```python
from build123d import *

# Parameters (mm, degrees)
SKETCH1_W           = 50.8
SKETCH1_H           = 6.6675
BOSS_EXTRUDE1_DEPTH = 44.45
CHAMFER1_SIZE       = 2.54
CHAMFER2_SIZE       = 2.54
SKETCH2_R           = 11.176
CUT_EXTRUDE1_DEPTH  = 44.45


with BuildPart() as part:
    # Sketch1 → Boss-Extrude1 (new body)
    with BuildSketch(Plane(origin=(0, 0, 0), x_dir=(1, 0, 0), z_dir=(0, 1, 0))):
        Polygon((0, 22.5425), (0, 15.875), (0, 9.2075), (0, 0), (41.275, 0), (41.275, 31.75), (0, 31.75), align=None)
        with Locations((-25.4, 19.20875)):
            Rectangle(SKETCH1_W, SKETCH1_H)
        with Locations((-25.4, 12.54125)):
            Rectangle(SKETCH1_W, SKETCH1_H)
    extrude(amount=BOSS_EXTRUDE1_DEPTH)

    # Chamfer1
    chamfer1_edges = [part.edges().sort_by_distance(p)[0] for p in [
        (0, 22.225, 0),
        (41.275, 22.225, -31.75),
        (41.275, 22.225, 0),
    ]]
    chamfer(chamfer1_edges, length=CHAMFER1_SIZE)

    # Chamfer2
    chamfer2_edges = [part.edges().sort_by_distance(p)[0] for p in [
        (0, 22.225, -31.75),
    ]]
    chamfer(chamfer2_edges, length=CHAMFER2_SIZE)

    # Sketch2 → Cut-Extrude1 (cut)
    with BuildSketch(Plane(origin=(0, 44.45, 0), x_dir=(1, 0, 0), z_dir=(0, 1, 0))):
        with Locations(Location((24.765, 15.875, 0), (0, 0, 270))):
            Circle(SKETCH2_R)
    extrude(amount=-CUT_EXTRUDE1_DEPTH, mode=Mode.SUBTRACT)


solid = part.part
```
Can you work these out from the model? Positions are in its coordinate system, mm. A direction names the side the tool comes from. Give positions to 0.01 mm unless a question says otherwise; leave off trailing zeros. Write each loop counter-clockwise with the first axis right and the second up, starting at its lowest first coordinate (ties: lowest second). Pieces come first, ordered by that corner, then holes. Notation, with made-up numbers: (48.25, 50.25) - (94.25, 50.25) arc R20 cw to (94.25, 56.25) - close; hole circle Ø5 at (-28.75, 2). An arc over 180 degrees is marked (long way). Write item = value, one per line. Start each with the question number.
1. On a 3-axis mill with a long thin cutter (end or side, diameter ignored), from which of +Z, -Z, +X, -X, +Y, -Y can I reach the whole of each face in a straight line? I mean faces 4 (the face through (39.987, 21.914, -30.498)), 5 (the face through (0, 22, -6)), 6 (the face through (-26, 22, -22.542)). Say none if no direction works.
2. Please list where these lines run through material, in increasing order: line 1 (Z direction, x = -14.5, y = 5); line 2 (X direction, y = 41, z = -9.5) (3 decimals); line 3 (Z direction, x = 32, y = 39).
3. Thinking about a two-plate mould opening in X: for faces 1 (the face through (20, 22, 0)), 2 (the face through (32.32, 22.54, -24.11)), 3 (the face through (-50.8, 22, -16)), which applies, released by +X, released by -X, zero draft, split by the parting line, or undercut?
4. For pin 1 (13.5 mm diameter, centred on x = -25.5, y = 27, fed in from +Z); pin 2 (5.5 mm diameter, centred on y = 22.5, z = -4.5, fed in from -X); pin 3 (22 mm diameter, centred on x = -27.5, y = 23, fed in from -Z); pin 4 (5 mm diameter, centred on x = -23, z = -5, fed in from +Y), each with a flat end and sliding along its axis, tell me the tip position at first contact or that it passes through.
5. Imagine slicing it at A-A (z = -17). Please give me the cut outline in (x, y) (3 decimals), and give its area (3 significant figures).
6. Imagine slicing it at B-B (x = 28). Please give me the cut outline in (y, z).
7. Imagine slicing it at D-D (x = -16). Please give me the cut outline in (y, z), and give its area (3 significant figures).
Worked answers:
q1.face_4 = -Z, +X, +Y, -Y
q1.face_5 = +Z, -X, +Y, -Y
q1.face_6 = -Z, -X, +Y, -Y
q2.line_1 = -22.54 to -9.21
q2.line_2 = -50.8 to 15.586, 33.944 to 41.275
q2.line_3 = -31.75 to -24.39, -7.36 to 0
q3.face_1 = zero draft
q3.face_2 = undercut
q3.face_3 = released by -X
q4.pin_1 = -9.21
q4.pin_2 = 0
q4.pin_3 = -22.54
q4.pin_4 = through
q5.outline = (-50.8, 0) - (13.646, 0) - (13.646, 44.45) - (-50.8, 44.45) - close; (35.884, 0) - (41.275, 0) - (41.275, 44.45) - (35.884, 44.45) - close
q5.area = 3,100 mm2
q6.outline = (0, -31.75) - (44.45, -31.75) - (44.45, -26.57) - (0, -26.57) - close; (0, -5.18) - (44.45, -5.18) - (44.45, 0) - (0, 0) - close
q7.outline = (0, -22.54) - (44.45, -22.54) - (44.45, -9.21) - (0, -9.21) - close
q7.area = 593 mm2
